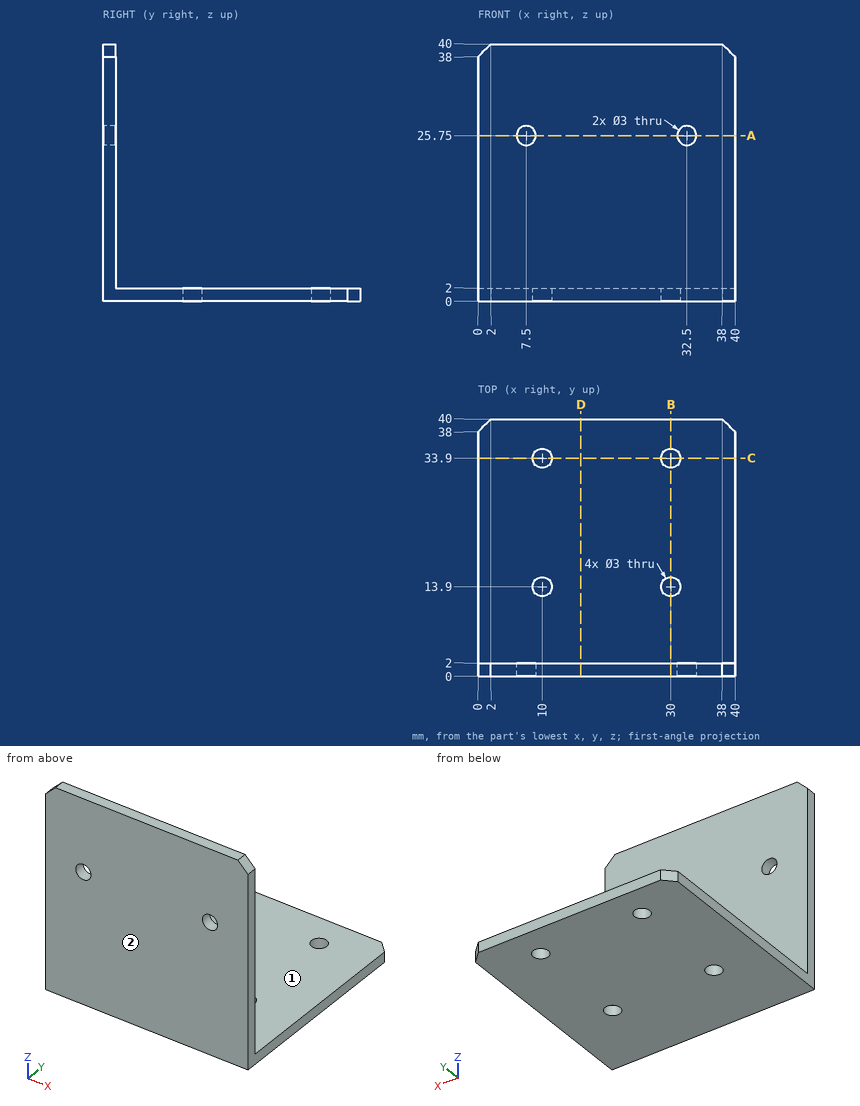
The figure shows three views and two pictorial views of one solid part (mm, origin at its lowest corner). Answer the questions. A direction names the side the tool comes from. Round coordinates to 2 decimals unless told otherwise and drop trailing zeros. Write each loop counter-clockwise with the first axis right and the second up, starting at its lowest first coordinate (ties: lowest second). Pieces come first, ordered by that corner, then holes. Notation, with made-up numbers: M 67,-6 L 123,-6 A17 cw 123,15 Z; hole C 21.25,85 d11. An arc over 180 degrees is marked long. Use a Markdown table: item, result.
1) Straight lines are drawn through the part: line 1 along X through (y, z) = (0.6, 25.75); line 2 along Z through (x, y) = (32.5, 1.1); line 3 along Y through (x, z) = (15.5, 14.5). For each, find the intervals that lie inside material, in ascending order. Write a range as [from, to].
Answers follow:
| item | result |
|---|---|
| line 1 | x = [0, 6], [9, 31], [34, 40] |
| line 2 | z = [0, 24.25], [27.25, 40] |
| line 3 | y = [0, 2] |
2) The part is cut by section C-C (y = 33.9). Write down the section's boundary in (x, z), plus the area to 3 significant figures.
Answers follow:
| item | result |
|---|---|
| outline | M 0,0 L 8.5,0 L 8.5,2 L 0,2 Z; M 11.5,0 L 28.5,0 L 28.5,2 L 11.5,2 Z; M 31.5,0 L 40,0 L 40,2 L 31.5,2 Z |
| area | 68.0 mm2 |
3) Flat-ended cylindrical pins translate along their axes: pin 1 (2.5 mm diameter, centred on x = 30, y = 13.9, fed in from +Z) (3 decimals); pin 2 (3.5 mm diameter, centred on x = 10, y = 13.9, fed in from +Z); pin 3 (4 mm diameter, centred on x = 5, z = 32, fed in from +Y). Find the tip coordinate at first contact, or state that the pin passes through.
Answers follow:
| item | result |
|---|---|
| pin 1 | passes through |
| pin 2 | stops at z = 2 |
| pin 3 | stops at y = 2 |
4) The part is cut by section A-A (z = 25.75). Write down the section's boundary in (x, y).
Answers follow:
| item | result |
|---|---|
| outline | M 0,0 L 6,0 L 6,2 L 0,2 Z; M 9,0 L 31,0 L 31,2 L 9,2 Z; M 34,0 L 40,0 L 40,2 L 34,2 Z |
5) A tool of negligible diameter and unlimited length cuts with its end or side. For the marked faces 1 and 2, from which of +Z, -Z, +X, -X, +Y, -Y can it reach the whole face along a straight path? Write none if from no direction.
Answers follow:
| item | result |
|---|---|
| face 1 | +Z, +X, -X, +Y |
| face 2 | +Z, -Z, +X, -X, -Y |
6) The part is cut by section B-B (x = 30). Write down the section's boundary in (y, z), plus the area to 3 significant figures.
Answers follow:
| item | result |
|---|---|
| outline | M 0,0 L 12.4,0 L 12.4,2 L 2,2 L 2,40 L 0,40 Z; M 15.4,0 L 32.4,0 L 32.4,2 L 15.4,2 Z; M 35.4,0 L 40,0 L 40,2 L 35.4,2 Z |
| area | 144 mm2 |
7) The part is cut by section D-D (x = 16). Write down the section's boundary in (y, z), plus the area to 3 significant figures.
Answers follow:
| item | result |
|---|---|
| outline | M 0,0 L 40,0 L 40,2 L 2,2 L 2,40 L 0,40 Z |
| area | 156 mm2 |
